Read the model definition and answer for the solid it produces. Units are mm, in the model's axes. A direction names the side the tool comes from. Give positions to 0.01 mm unless a question says otherwise; leave off trailing zeros. Loops run counter-clockwise (first coordinate to the right, second up) from the corner with the lowest first, then second, coordinate; pieces in that order, holes last. Notation, with made-up numbers: M -31,57.5 L 1,57.5 A25 ccw 1,69.5 Z; hole C 85,32.25 d10. An arc over 180 degrees is marked long. Return JSON: item names as keys, results as strings. Group by question number.
```python
from build123d import *

# Parameters (mm, degrees)
CROQUIS1_W              = 16
CROQUIS1_H              = 11.5
CROQUIS1_R              = 2.5
CROQUIS1_H_2            = 3
SALIENTE_EXTRUIR1_DEPTH = 5
CROQUIS4_W              = 16
CROQUIS4_H              = 3
SALIENTE_EXTRUIR3_DEPTH = 25
CROQUIS6_R              = 1
CORTAR_EXTRUIR1_DEPTH   = 25
CROQUIS7_W              = 1
CROQUIS7_H              = 30
CORTAR_EXTRUIR2_DEPTH   = 25


with BuildPart() as part:
    # Croquis1 → Saliente-Extruir1 (new body)
    # profile 1 of 2: a face of its own
    with BuildSketch(Plane(origin=(0, 0, 0), x_dir=(1, 0, 0), z_dir=(0, 1, 0))):
        Rectangle(CROQUIS1_W, CROQUIS1_H)
        with Locations(Location((0, 0, 0), (0, 0, 270))):
            Circle(CROQUIS1_R, mode=Mode.SUBTRACT)
    # profile 2 of 2: a face of its own
    with BuildSketch(Plane(origin=(0, 0, 0), x_dir=(1, 0, 0), z_dir=(0, 1, 0))):
        with Locations((0, -7.25)):
            Rectangle(CROQUIS1_W, CROQUIS1_H_2)
    extrude(amount=SALIENTE_EXTRUIR1_DEPTH)

    # Croquis4 → Saliente-Extruir3 (add)
    with BuildSketch(Plane(origin=(0, 5, 0), x_dir=(1, 0, 0), z_dir=(0, 1, 0))):
        with Locations((0, -7.25)):
            Rectangle(CROQUIS4_W, CROQUIS4_H)
    extrude(amount=SALIENTE_EXTRUIR3_DEPTH)

    # Croquis6 → Cortar-Extruir1 (cut)
    with BuildSketch(Plane.XY.offset(8.75)):
        with Locations((-4, 22.38)):
            Circle(CROQUIS6_R)
        with Locations((-4, 13)):
            Circle(CROQUIS6_R)
    extrude(amount=-CORTAR_EXTRUIR1_DEPTH, mode=Mode.SUBTRACT)

    # Croquis7 → Cortar-Extruir2 (cut)
    with BuildSketch(Plane.XY.offset(8.75)):
        with Locations((7.5, 15)):
            Rectangle(CROQUIS7_W, CROQUIS7_H)
    extrude(amount=-CORTAR_EXTRUIR2_DEPTH, mode=Mode.SUBTRACT)


solid = part.part
```
1. For faces 1 (the flat face through (-1, 15, 8.75)), 2 (the flat face through (-1, 17, 5.75)), determine the directions among +Z, -Z, +X, -X, +Y, -Y from which every point of the face is accessible in a straight line to the end or side of a thin tool.
2. The mould has two halves that part along X. Classify faces 3 (the flat face through (-8, 8, 6)), 4 (the cylindrical face through (-2.44, 2.46, -0.54)), 5 (the flat face through (-1, 0, 3)): +X half, -X half, draft (parallel to the pull), parting line (faces both ways), or undercut.
3. Find section A-A (z = 0). Write down the section's boundary in (x, y).
4. Find section C-C (y = 22.38). Write down the section's boundary in (x, z), and give its area (3 significant figures).
5. Flat-ended cylindrical pins translate along their axes: P1, Ø1.8, axis at x = -4, y = 13, coming from the +Z side; P2, Ø3, axis at x = -5, z = 0.5, coming from the +Y side. Find the tip coordinate at first contact, or state that the pin passes through.
6. Straight lines are drawn through the part: line 1 along Y through (x, z) = (-4, 8); line 2 along X through (y, z) = (2.1, 0); line 3 along Y through (x, z) = (-1.75, -4.5). For each, find the intervals that lie inside material, in ascending order.
7. Find section D-D (x = 0). Write down the section's boundary in (y, z), and give its area (4 significant figures).
8. Find section B-B (x = -4). Write down the section's boundary in (y, z).
Result:
{
 "1": {"face 1": "+Z, +X, -X, +Y, -Y", "face 2": "-Z, +X, -X, +Y"},
 "2": {"face 3": "-X half", "face 4": "undercut", "face 5": "draft"},
 "3": {"outline": "M -8,0 L -2.5,0 L -2.5,5 L -8,5 Z; M 2.5,0 L 7,0 L 7,5 L 2.5,5 Z"},
 "4": {"outline": "M -8,5.75 L -5,5.75 L -5,8.75 L -8,8.75 Z; M -3,5.75 L 7,5.75 L 7,8.75 L -3,8.75 Z", "area": "39.0 mm2"},
 "5": {"P1": "passes through", "P2": "stops at y = 5"},
 "6": {"line 1": "y = 0 to 12, 14 to 21.38, 23.38 to 30", "line 2": "x = -8 to -2.5, 2.5 to 7", "line 3": "y = 0 to 5"},
 "7": {"outline": "M 0,-5.75 L 5,-5.75 L 5,-2.5 L 0,-2.5 Z; M 0,2.5 L 5,2.5 L 5,5.75 L 30,5.75 L 30,8.75 L 0,8.75 Z", "area": "122.5 mm2"},
 "8": {"outline": "M 0,-5.75 L 5,-5.75 L 5,5.75 L 12,5.75 L 12,8.75 L 0,8.75 Z; M 14,5.75 L 21.38,5.75 L 21.38,8.75 L 14,8.75 Z; M 23.38,5.75 L 30,5.75 L 30,8.75 L 23.38,8.75 Z"}
}
